Input: part model. Units: mm. Frame: model coordinates. Face numbers are marked on the shaded views. A direction names the side the tool comes from. Give positions to 0.01 mm unless a question says otherwise; leave off trailing zeros. Order: outer loops, then holes, each group sorted by start corner. A loop starts at its lowest first (then second) coordinate and runs counter-clockwise, first axis right, second up. Notation, with made-up numbers: (35, -34.75) - (42, -34.75) arc R27 ccw to (42, -15.75) - close; hole circle Ø9 at (79, 41.5). An arc over 180 degrees is marked (long way). Answer in a Markdown table with one row per item. Add a question column.
1. Ray query, line 1 (X direction, y = -12, z = 1.5); line 2 (X direction, y = 8.5, z = 0.5); line 3 (X direction, y = -4.5, z = 8). Return the intervals inside material, ascending. Write a range as [from, to].
2. Section query A-A on z = 5.25. Return loops of the section in (x, y), and give its area (3 significant figures).
3. Section query D-D on x = -15. Return loops of the section in (y, z), and give its area (3 significant figures).
4. Mould query, pull axis Y, two halves, no side actions, for the marked faces 4, 5 and 6. Classes: released by +Y, released by -Y, zero draft, split by the parting line, or undercut.
5. Contact query for flat-ended pins moving along their axis: pin 1 (6 mm diameter, centred on x = 10, z = 6.5, fed in from +Y); pin 2 (9.5 mm diameter, centred on y = -3.5, z = 3.5, fed in from +X); pin 3 (7 mm diameter, centred on x = 16.5, y = 0.5, fed in from +Z). Output: stop coordinate, or through.
6. Section query C-C on x = 6. Return loops of the section in (y, z), and give its area (3 significant figures).
7. Section query B-B on y = -12. Return loops of the section in (x, z).
8. Access query for the marked faces 1, 2 and 3. Directions: +Z, -Z, +X, -X, +Y, -Y. A direction counts if a zero-diameter tool reaches every point of the face in a straight line with its end or side. Return the directions, or none.
```python
from build123d import *

# Parameters (mm, degrees)
F0_W      = 34.9287392313
F0_H      = 32
F0_W_2    = 32.1578574658
F0_H_2    = 29.2369164526
F0_W_3    = 31.648522869
F0_W_4    = 26
F0_H_3    = 26
F0_R      = 0.092316022
F0_R_2    = 0.0979069207
F0_R_3    = 0.103754176
F0_R_4    = 0.0980954436
F0_R_5    = 0.0966883049
F0_R_6    = 0.10446749
F0_R_7    = 0.1013580247
F0_W_5    = 23
F0_H_4    = 23
F1_DEPTH  = 10
F2_DEPTH  = 2
F3_DEPTH  = 12
F4_R      = 1.1151905594
F5_DEPTH  = 51
F4_R_2    = 2.9667518112
F6_DEPTH  = 8
F7_SIZE   = 0.7
F8_DEPTH  = 1
F10_R     = 0.4707857642
F11_DEPTH = 4


with BuildPart() as f1:
    # F0 (on Top) → F1 (new body)
    with BuildSketch(Plane.XY):
        with Locations((-15.8242614345, 0)):
            Rectangle(F0_W, F0_H)
        with Locations((-15.8211605012, 0.0195009634)):
            Rectangle(F0_W_2, F0_H_2, mode=Mode.SUBTRACT)
        with Locations((17.4643696156, 0)):
            Rectangle(F0_W_3, F0_H)
        with Locations((16.7290959507, 0)):
            Rectangle(F0_W_4, F0_H_3, mode=Mode.SUBTRACT)
        with Locations((-15.8211605012, 0.0195009634)):
            Rectangle(F0_W_2, F0_H_2)
        with Locations((-16.4775699377, -0.2384704421)):
            Circle(F0_R, mode=Mode.SUBTRACT)
        with Locations((-16.1935091019, -0.2361788647)):
            Circle(F0_R_2, mode=Mode.SUBTRACT)
        with Locations((-16.6078936309, 0.000503382)):
            Circle(F0_R_3, mode=Mode.SUBTRACT)
        with Locations((-16.3381490856, 0)):
            Circle(F0_R_4, mode=Mode.SUBTRACT)
        with Locations((-16.4667107165, 0.2449084714)):
            Circle(F0_R_5, mode=Mode.SUBTRACT)
        with Locations((-16.1935091019, 0.2444714482)):
            Circle(F0_R_6, mode=Mode.SUBTRACT)
        with Locations((-16.0595625639, 0)):
            Circle(F0_R_7, mode=Mode.SUBTRACT)
        with Locations((16.7290959507, 0)):
            Rectangle(F0_W_4, F0_H_3)
        with Locations((16.7408101037, 0.1883851588)):
            Rectangle(F0_W_5, F0_H_4, mode=Mode.SUBTRACT)
        with Locations((16.7408101037, 0.1883851588)):
            Rectangle(F0_W_5, F0_H_4)
        with Locations((-16.1935091019, 0.2444714482)):
            Circle(F0_R_6)
        with Locations((-16.6078936309, 0.000503382)):
            Circle(F0_R_3)
        with Locations((-16.0595625639, 0)):
            Circle(F0_R_7)
        with Locations((-16.3381490856, 0)):
            Circle(F0_R_4)
        with Locations((-16.1935091019, -0.2361788647)):
            Circle(F0_R_2)
        with Locations((-16.4667107165, 0.2449084714)):
            Circle(F0_R_5)
        with Locations((-16.4775699377, -0.2384704421)):
            Circle(F0_R)
    extrude(amount=-F1_DEPTH)

    # F0 (on Top) → F2 (join)
    with BuildSketch(Plane.XY):
        with Locations((-15.8242614345, 0)):
            Rectangle(F0_W, F0_H)
        with Locations((-15.8211605012, 0.0195009634)):
            Rectangle(F0_W_2, F0_H_2, mode=Mode.SUBTRACT)
    extrude(amount=F2_DEPTH)

    # F0 (on Top) → F3 (join)
    with BuildSketch(Plane.XY):
        with Locations((16.7290959507, 0)):
            Rectangle(F0_W_4, F0_H_3)
        with Locations((16.7408101037, 0.1883851588)):
            Rectangle(F0_W_5, F0_H_4, mode=Mode.SUBTRACT)
    extrude(amount=F3_DEPTH)

    # F4 (on face) → F5 (cut)
    with BuildSketch(Plane.YZ.offset(33.2886310501)):
        with Locations((0, -5.1095909439)):
            Circle(F4_R)
    extrude(amount=-F5_DEPTH, mode=Mode.SUBTRACT)

    # F4 (on face) → F6 (join)
    with BuildSketch(Plane.YZ.offset(33.2886310501)):
        with Locations((0, -5.1095909439)):
            Circle(F4_R_2)
        with Locations((0, -5.1095909439)):
            Circle(F4_R, mode=Mode.SUBTRACT)
    extrude(amount=F6_DEPTH)

    # F7
    f7_edges = [f1.edges().sort_by_distance(p)[0] for p in [
        (41.288631, -2.966752, -5.109591),
    ]]
    chamfer(f7_edges, length=F7_SIZE)

    # F0 (on Top) → F8 (cut)
    with BuildSketch(Plane.XY):
        with Locations((-16.4667107165, 0.2449084714)):
            Circle(F0_R_5)
        with Locations((-16.1935091019, 0.2444714482)):
            Circle(F0_R_6)
        with Locations((-16.0595625639, 0)):
            Circle(F0_R_7)
        with Locations((-16.1935091019, -0.2361788647)):
            Circle(F0_R_2)
        with Locations((-16.4775699377, -0.2384704421)):
            Circle(F0_R)
        with Locations((-16.6078936309, 0.000503382)):
            Circle(F0_R_3)
        with Locations((-16.3381490856, 0)):
            Circle(F0_R_4)
    extrude(amount=-F8_DEPTH, mode=Mode.SUBTRACT)

    # F10 (on offset) → F11 (cut)
    with BuildSketch(Plane.XY.offset(-1)):
        with Locations((-16.3349304348, -0.0002074475)):
            Circle(F10_R)
    extrude(amount=-F11_DEPTH, mode=Mode.SUBTRACT)


solid = f1.part
```
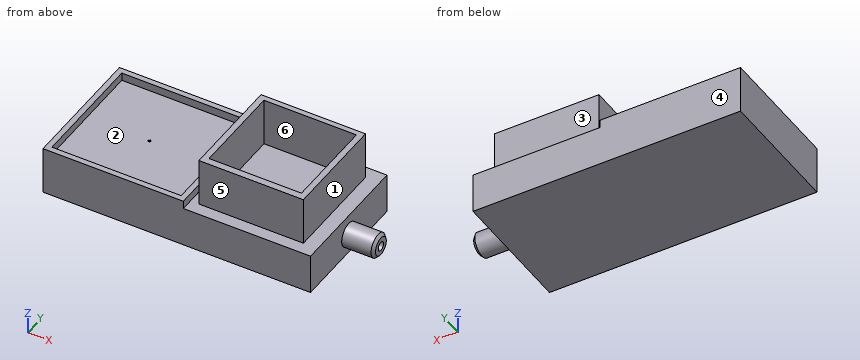
Answer:
| question | item | result |
|---|---|---|
| 1 | line 1 | x = [-33.29, -31.9], [0.26, 1.64], [3.73, 29.73] |
| 1 | line 2 | x = [-33.29, -31.9], [0.26, 1.64], [3.73, 5.24], [28.24, 29.73] |
| 1 | line 3 | x = [3.73, 5.24], [28.24, 29.73] |
| 2 | outline | (3.73, -13) - (29.73, -13) - (29.73, 13) - (3.73, 13) - close; hole (5.24, -11.31) - (28.24, -11.31) - (28.24, 11.69) - (5.24, 11.69) - close |
| 2 | area | 147 mm² |
| 3 | outline | (-16, -10) - (16, -10) - (16, 2) - (14.64, 2) - (14.64, 0) - (-14.6, 0) - (-14.6, 2) - (-16, 2) - close; hole circle Ø2.23 at (0, -5.11) |
| 3 | area | 322 mm² |
| 4 | face 4 | released by +Y |
| 4 | face 5 | released by -Y |
| 4 | face 6 | undercut |
| 5 | pin 1 | stops at y = 13 |
| 5 | pin 2 | stops at x = 33.29 |
| 5 | pin 3 | stops at z = 0 |
| 6 | outline | (-16, -10) - (16, -10) - (16, 0) - (13, 0) - (13, 12) - (11.69, 12) - (11.69, 0) - (-11.31, 0) - (-11.31, 12) - (-13, 12) - (-13, 0) - (-16, 0) - close; hole circle Ø2.23 at (0, -5.11) |
| 6 | area | 352 mm² |
| 7 | outline | (-33.29, -10) - (33.29, -10) - (33.29, 0) - (29.73, 0) - (29.73, 12) - (3.73, 12) - (3.73, 0) - (1.64, 0) - (1.64, 2) - (0.26, 2) - (0.26, 0) - (-31.9, 0) - (-31.9, 2) - (-33.29, 2) - close |
| 8 | face 1 | +Z, +X, +Y, -Y |
| 8 | face 2 | +Z |
| 8 | face 3 | +Z, +X, +Y |
